from build123d import *

# Parameters (mm, degrees)
SZKIC1_R                    = 1.5
DODANIE_WYCI_GNI_CIE1_DEPTH = 2
SZKIC2_R                    = 1.5
DODANIE_WYCI_GNI_CIE2_DEPTH = 3
WYTNIJ_WYCI_GNI_CIE1_DEPTH  = 2.5
SFAZOWANIE1_SIZE            = 3
SFAZOWANIE2_SIZE            = 2
SFAZOWANIE3_SIZE            = 0.5


with BuildPart() as part:
    # Szkic1 → Dodanie-wyciągnięcie1 (new body)
    with BuildSketch(Plane.XY):
        with BuildLine():
            Line((-4, 0), (-4, 45))
            ThreePointArc((-4, 45), (0, 49), (4, 45))
            Line((4, 45), (4, 0))
            ThreePointArc((4, 0), (0, -4), (-4, 0))
        make_face()
        Circle(SZKIC1_R, mode=Mode.SUBTRACT)
        with BuildLine():
            Line((1.5, 45), (1.5, 15))
            ThreePointArc((1.5, 15), (0, 13.5), (-1.5, 15))
            Line((-1.5, 15), (-1.5, 45))
            ThreePointArc((-1.5, 45), (0, 46.5), (1.5, 45))
        make_face(mode=Mode.SUBTRACT)
    extrude(amount=DODANIE_WYCI_GNI_CIE1_DEPTH)

    # Szkic2 → Dodanie-wyciągnięcie2 (add)
    with BuildSketch(Plane.XY.offset(2)):
        with BuildLine():
            Line((-4, 9), (4, 9))
            Line((4, 9), (4, 0))
            ThreePointArc((4, 0), (0, -4), (-4, 0))
            Line((-4, 0), (-4, 9))
        make_face()
        Circle(SZKIC2_R, mode=Mode.SUBTRACT)
    extrude(amount=DODANIE_WYCI_GNI_CIE2_DEPTH)

    # Szkic3 → Wytnij-wyciągnięcie1 (cut)
    with BuildSketch(Plane(origin=(0, 0, 0), x_dir=(-1, 0, 0), z_dir=(0, 0, -1))):
        with BuildLine():
            Line((-4, 7), (4, 7))
            Line((4, 7), (4, 0))
            ThreePointArc((4, 0), (0, -4), (-4, 0))
            Line((-4, 0), (-4, 7))
        make_face()
    extrude(amount=-WYTNIJ_WYCI_GNI_CIE1_DEPTH, mode=Mode.SUBTRACT)

    # Sfazowanie1
    sfazowanie1_edges = [part.edges().sort_by_distance(p)[0] for p in [
        (0, 9, 2),
    ]]
    chamfer(sfazowanie1_edges, length=SFAZOWANIE1_SIZE - 0.0001)  # a hair under: the kernel refuses the full size

    # Sfazowanie2
    sfazowanie2_edges = [part.edges().sort_by_distance(p)[0] for p in [
        (0, 7, 0),
    ]]
    chamfer(sfazowanie2_edges, length=SFAZOWANIE2_SIZE)

    # Sfazowanie3
    sfazowanie3_edges = [part.edges().sort_by_distance(p)[0] for p in [
        (0, 7, 2.5),
    ]]
    chamfer(sfazowanie3_edges, length=SFAZOWANIE3_SIZE - 0.0001)  # a hair under: the kernel refuses the full size


solid = part.part
Part model, mm, in its own coordinate system. A direction names the side the tool comes from. Coordinates: 2 decimals unless noted, no trailing zeros. Order: outer loops, then holes, each group sorted by start corner. A loop starts at its lowest first (then second) coordinate and runs counter-clockwise, first axis right, second up. Notation, with made-up numbers: M -27,58.5 L 25,58.5 A22 ccw 25,90.5 Z; hole C -28,-33.75 d10. An arc over 180 degrees is marked long. One line per question, with ' | ' between items.
Q1. Slice it at B-B (y = 26). Give the cut face in (x, z).
A:
outline: M -4,0 L -1.5,0 L -1.5,2 L -4,2 Z; M 1.5,0 L 4,0 L 4,2 L 1.5,2 Z
Q2. Slice it at C-C (z = 0.45). Give the cut face in (x, y).
A:
outline: M -4,8.55 L 4,8.55 L 4,45 A4 ccw -4,45 Z; hole M -1.5,15 A1.5 ccw 1.5,15 L 1.5,45 A1.5 ccw -1.5,45 Z
Q3. 3-axis set-ups, long thin cutter, end or side, ignore diameter. For faces 4 (the face through (0, 2, 2.5)), 5 (the face through (1.5, 30, 1)), 6 (the face through (2, 31, 2)): which of +Z, -Z, +X, -X, +Y, -Y reach the whole face in a straight line?
A:
face 4: -Z, +X, -X, -Y | face 5: +Z, -Z | face 6: +Z, +X, -X, +Y
Q4. Pin check, flat tips, straight feed: P1, Ø1.8, axis at x = 0, y = 0, coming from the -Z side; P2, Ø2, axis at x = -1.5, z = 2, coming from the -Y side; P3, Ø4, axis at x = 0.5, y = 31.5, coming from the +Z side; P4, Ø1, axis at x = 3, z = 4, coming from the +Y side. Stop position of each tip, or through.
A:
P1: passes through | P2: stops at y = -3.95 | P3: stops at z = 2 | P4: stops at y = 10.5
Q5. Slice it at A-A (x = 0). Count the separate pieces of the cut face and the enclosed holes in it, and give its area (3 significant figures).
A:
separate pieces: 3 | enclosed holes: 0 | area: 46.6 mm^2
Q6. Two-plate mould, pull along Y, no slides. Class faces 1 (the face through (2, 29, 0)), 2 (the face through (-1.5, 0.07, 3.73)), 3 (the face through (0, 49, 1)): +Y half, -Y half, draft (parallel to the pull), parting line (faces both ways), or undercut.
A:
face 1: draft | face 2: undercut | face 3: +Y half
Q7. Drill centre lines: line 1 (X direction, y = 31.5, z = 0.45); line 2 (Z direction, x = -2.75, y = 38); line 3 (Z direction, x = 2, y = 3). Where is each one in solid material? Low to high.
A:
line 1: x = -4 to -1.5, 1.5 to 4 | line 2: z = 0 to 2 | line 3: z = 2.5 to 5
